from build123d import *

# Parameters (mm, degrees)
EXTRUS_O_PRINCIPAL_DEPTH                            = 50
REBAIXO_CAMISA_DEPTH                                = 36.5
FILETE_ALIVIO_REBAIXO_R                             = 8
ESBO_O2_3_R                                         = 30
FURO_EIXO_DEPTH                                     = 181.048651344
CORTE_EXTRUS_O1_START                               = -36.5
ESBO_O2_4_R                                         = 37.5
CORTE_EXTRUS_O1_DEPTH                               = 2
ESCAREADO_PARA_PARAFUSO_ALLEN_SEXTAVADO_D           = 17
ESCAREADO_PARA_PARAFUSO_ALLEN_SEXTAVADO_CSINK_D     = 33.6
ESCAREADO_PARA_PARAFUSO_ALLEN_SEXTAVADO_CSINK_ANGLE = 90


with BuildPart() as part:
    # Sketch2 → EXTRUSÃO PRINCIPAL (new body)
    with BuildSketch(Plane.XY):
        with BuildLine():
            Line((-127.578119637, 46.051076804), (-149.014261062, 51))
            Line((-149.014261062, 51), (-151.136776123, 10.5))
            Line((-151.136776123, 10.5), (-126.552927997, -37.748518598))
            ThreePointArc((-126.552927997, -37.748518598), (-106.644110754, -60.251342967), (-78.321881111, -70.280770499))
            Line((-78.321881111, -70.280770499), (78.489629635, -84))
            ThreePointArc((78.489629635, -84), (94.087674002, -81.159159507), (106.059471738, -70.764669536))
            ThreePointArc((106.059471738, -70.764669536), (127.499968454, -0.089689786), (106.158925464, 70.615384615))
            ThreePointArc((106.158925464, 70.615384615), (95.349660705, 80.44297202), (81.180354766, 84))
            Line((81.180354766, 84), (-58.932234692, 84))
            ThreePointArc((-58.932234692, 84), (-73.932234692, 79.980762114), (-84.912996806, 69))
            Line((-84.912996806, 69), (-88.302967145, 63.128399137))
            ThreePointArc((-88.302967145, 63.128399137), (-105.1249152, 48.114236459), (-127.578119637, 46.051076804))
        make_face()
    extrude(amount=EXTRUS_O_PRINCIPAL_DEPTH)

    # Esboço2 → REBAIXO CAMISA (cut)
    with BuildSketch(Plane(origin=(0, 0, 0), x_dir=(-1, 0, 0), z_dir=(0, 0, -1))):
        with BuildLine():
            Line((-48.331774145, 55.581801869), (42.321943382, 63.512974459))
            ThreePointArc((42.321943382, 63.512974459), (51.081263611, 60.751171399), (55.322148672, 52.604506995))
            Line((55.322148672, 52.604506995), (63.253321262, -38.049210532))
            ThreePointArc((63.253321262, -38.049210532), (60.491518202, -46.808530761), (52.344853798, -51.049415822))
            Line((52.344853798, -51.049415822), (-38.308863729, -58.980588412))
            ThreePointArc((-38.308863729, -58.980588412), (-47.068183958, -56.218785352), (-51.309069019, -48.072120948))
            Line((-51.309069019, -48.072120948), (-59.240241609, 42.581596579))
            ThreePointArc((-59.240241609, 42.581596579), (-56.478438549, 51.340916808), (-48.331774145, 55.581801869))
        make_face()
    extrude(amount=-REBAIXO_CAMISA_DEPTH, mode=Mode.SUBTRACT)

    # FILETE ALIVIO REBAIXO
    filete_alivio_rebaixo_edges = [part.edges().sort_by_distance(p)[0] for p in [
        (3.004915382, 59.547388164, 0),
        (-51.081263611, 60.751171399, 0),
        (-59.287734967, 7.277648231, 0),
        (56.478438549, 51.340916808, 0),
        (55.274655314, -2.745262185, 0),
        (47.068183958, -56.218785352, 0),
        (-7.017995034, -55.015002117, 0),
        (-60.491518202, -46.808530761, 0),
    ]]
    fillet(filete_alivio_rebaixo_edges, radius=FILETE_ALIVIO_REBAIXO_R)

    # Esboço2<3> → FURO EIXO (cut, through all)
    with BuildSketch(Plane(origin=(0, 0, 0), x_dir=(-1, 0, 0), z_dir=(0, 0, -1))):
        with Locations((2.006539826, 2.266193023)):
            Circle(ESBO_O2_3_R)
    extrude(amount=-FURO_EIXO_DEPTH, mode=Mode.SUBTRACT)

    # Esboço2<4> → Corte-extrusão1 (cut)
    with BuildSketch(Plane(origin=(0, 0, 0), x_dir=(-1, 0, 0), z_dir=(0, 0, -1)).offset(CORTE_EXTRUS_O1_START)):
        with Locations((2.006539826, 2.266193023)):
            Circle(ESBO_O2_4_R)
    extrude(amount=-CORTE_EXTRUS_O1_DEPTH, mode=Mode.SUBTRACT)

    # Escareado para parafuso Allen sextavado escareado de M161 (through all)
    with Locations(Plane.XY.offset(50)):
        with Locations((-39.731656473, 47.225236318), (42.952503468, 39.99130967), (-46.965583121, -35.458923623), (35.71857682, -42.692850271)):
            CounterSinkHole(ESCAREADO_PARA_PARAFUSO_ALLEN_SEXTAVADO_D / 2, ESCAREADO_PARA_PARAFUSO_ALLEN_SEXTAVADO_CSINK_D / 2, counter_sink_angle=ESCAREADO_PARA_PARAFUSO_ALLEN_SEXTAVADO_CSINK_ANGLE)


solid = part.part
Geometry check sheet. Reference: the model listing, model coordinates, mm. A direction names the side the tool comes from. Coordinates: 2 decimals unless noted, no trailing zeros. Order: outer loops, then holes, each group sorted by start corner. A loop starts at its lowest first (then second) coordinate and runs counter-clockwise, first axis right, second up. Notation, with made-up numbers: (15, 48) -> (57, 48) arc R19 cw to (57, 71) -> close; hole circle Ø7 at (63.5, 6). An arc over 180 degrees is marked (long way). Use a Markdown table: item, result. Add a question column.
1. Cross-section at B-B (x = 91.5). Enter the section's corners in (y, z), and give its area (3 significant figures).
2. Material ranges on L1, parallel to Y at x = -50.5, z = 47.5; L2, parallel to Y at x = -43.5, z = 29; L3, parallel to Y at x = 4.5, z = 11, recorded low to high.
3. Set-up check for faces 1 (the face through (34.73, 36.58, 42.1)), 2 (the face through (57.73, -2.32, 2.28)): record each of +Z, -Z, +X, -X, +Y, -Y from which the full face is reachable in a straight line by a thin tool's end or side.
4. Go/stop test with flat-tipped pins: pin 1 Ø4 at (x, z) = (17.5, 31) entering from -Y; pin 2 Ø10 at (y, z) = (18, 8) entering from -X; pin 3 Ø22 at (x, y) = (-46.97, -35.46) entering from +Z. Record where each tip stops, or that it passes through.
5. Cross-section at A-A (z = 11). Enter the section's corners in (x, y), and give its area (3 significant figures).
6. Mould release check, pull along Y, two halves, no side actions. Record for faces 3 (the face through (-1.014, -77.044, 24.65)), 4 (the face through (-14, 38, 50)), 5 (the face through (-33.467, 52.97, 39.064)): pulls with the +Y half, pulls with the -Y half, needs draft (parallel to the pull), parting line crosses it, or undercut.
7. Cross-section at C-C (x = -117.5). Enter the section's corners in (y, z), and give its area (3 significant figures).
Filled sheet:
| question | item | result |
|---|---|---|
| 1 | outline | (-82.26, 0) -> (82.17, 0) -> (82.17, 50) -> (-82.26, 50) -> close |
| 1 | area | 8,220 mm2 |
| 2 | L1 | -72.71 to -49.32, -21.6 to 37.82, 56.63 to 84 |
| 2 | L2 | -73.33 to -51.82, 63.56 to 84 |
| 2 | L3 | -77.53 to -56.02, 59.42 to 84 |
| 3 | face 1 | +Z |
| 3 | face 2 | -Z |
| 4 | pin 1 | y = -78.84 |
| 4 | pin 2 | x = -151.01 |
| 4 | pin 3 | z = 44.2 |
| 5 | outline | (-151.14, 10.5) -> (-126.55, -37.75) arc R60 ccw to (-78.32, -70.28) -> (78.49, -84) arc R30 ccw to (106.06, -70.76) arc R127.5 ccw to (106.16, 70.62) arc R30 ccw to (81.18, 84) -> (-58.93, 84) arc R30 ccw to (-84.91, 69) -> (-88.3, 63.13) arc R36 cw to (-127.58, 46.05) -> (-149.01, 51) -> close; hole (-63.25, -38.05) arc R12 ccw to (-52.34, -51.05) -> (38.31, -58.98) arc R12 ccw to (51.31, -48.07) -> (59.24, 42.58) arc R12 ccw to (48.33, 55.58) -> (-42.32, 63.51) arc R12 ccw to (-55.32, 52.6) -> close |
| 5 | area | 25,600 mm2 |
| 6 | face 3 | pulls with the -Y half |
| 6 | face 4 | needs draft |
| 6 | face 5 | undercut |
| 7 | outline | (-50.86, 0) -> (45.18, 0) -> (45.18, 50) -> (-50.86, 50) -> close |
| 7 | area | 4,800 mm2 |
